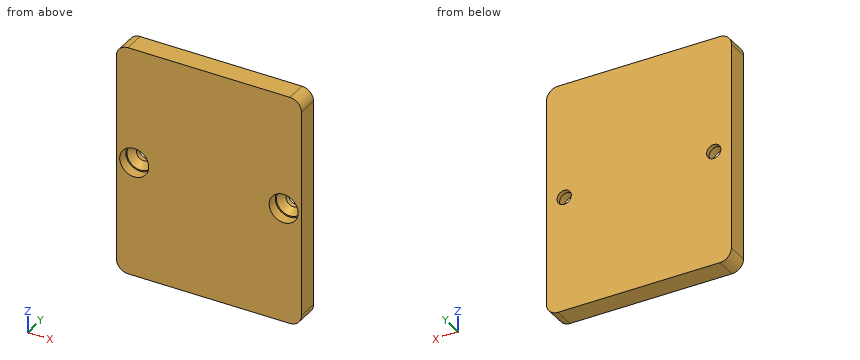
from build123d import *

# Parameters (mm, degrees)
SKETCH1_R                                       = 1.5
BOSS_EXTRUDE1_DEPTH                             = 2.5
CSK_FOR_M3_FLAT_HEAD_MACHINE_SCREW1_D           = 3.4
CSK_FOR_M3_FLAT_HEAD_MACHINE_SCREW1_DEPTH       = 10
CSK_FOR_M3_FLAT_HEAD_MACHINE_SCREW1_CSINK_D     = 6.3
CSK_FOR_M3_FLAT_HEAD_MACHINE_SCREW1_CSINK_ANGLE = 90
CSK_FOR_M3_FLAT_HEAD_MACHINE_SCREW1_TIP         = 1.021463052
BOSS_EXTRUDE2_START                             = 2.5
SKETCH4_R                                       = 3.45
BOSS_EXTRUDE2_DEPTH                             = 2.5


with BuildPart() as part:
    # Sketch1 → Boss-Extrude1 (new body)
    with BuildSketch(Plane(origin=(0, 0, 0), x_dir=(1, 0, 0), z_dir=(0, 1, 0))):
        with BuildLine():
            Line((-19.25, -27.5), (19.25, -27.5))
            ThreePointArc((19.25, -27.5), (21.194543648, -26.694543648), (22, -24.75))
            Line((22, -24.75), (22, 24.75))
            ThreePointArc((22, 24.75), (21.194543648, 26.694543648), (19.25, 27.5))
            Line((19.25, 27.5), (-19.25, 27.5))
            ThreePointArc((-19.25, 27.5), (-21.194543648, 26.694543648), (-22, 24.75))
            Line((-22, 24.75), (-22, -24.75))
            ThreePointArc((-22, -24.75), (-21.194543648, -26.694543648), (-19.25, -27.5))
        make_face()
        with Locations(Location((-17.78, 0, 0), (0, 0, 270))):
            Circle(SKETCH1_R, mode=Mode.SUBTRACT)
        with Locations(Location((17.78, 0, 0), (0, 0, 90))):
            Circle(SKETCH1_R, mode=Mode.SUBTRACT)
    extrude(amount=BOSS_EXTRUDE1_DEPTH)

    # CSK for M3 Flat Head Machine Screw1
    with Locations(Plane(origin=(0, 0, 0), x_dir=(-1, 0, 0), z_dir=(0, -1, 0))):
        with Locations((-17.78, 0), (17.78, 0)):
            CounterSinkHole(CSK_FOR_M3_FLAT_HEAD_MACHINE_SCREW1_D / 2, CSK_FOR_M3_FLAT_HEAD_MACHINE_SCREW1_CSINK_D / 2, depth=CSK_FOR_M3_FLAT_HEAD_MACHINE_SCREW1_DEPTH, counter_sink_angle=CSK_FOR_M3_FLAT_HEAD_MACHINE_SCREW1_CSINK_ANGLE)
            with Locations((0, 0, -(CSK_FOR_M3_FLAT_HEAD_MACHINE_SCREW1_DEPTH + CSK_FOR_M3_FLAT_HEAD_MACHINE_SCREW1_TIP / 2))):  # 118° drill point
                Cone(0, CSK_FOR_M3_FLAT_HEAD_MACHINE_SCREW1_D / 2, CSK_FOR_M3_FLAT_HEAD_MACHINE_SCREW1_TIP, mode=Mode.SUBTRACT)

    # Sketch4 → Boss-Extrude2 (add)
    with BuildSketch(Plane.XZ.offset(BOSS_EXTRUDE2_START)):
        with BuildLine():
            Line((-22, 24.75), (-22, -24.75))
            ThreePointArc((-22, -24.75), (-21.194543648, -26.694543648), (-19.25, -27.5))
            Line((-19.25, -27.5), (19.25, -27.5))
            ThreePointArc((19.25, -27.5), (21.194543648, -26.694543648), (22, -24.75))
            Line((22, -24.75), (22, 24.75))
            ThreePointArc((22, 24.75), (21.194543648, 26.694543648), (19.25, 27.5))
            Line((19.25, 27.5), (-19.25, 27.5))
            ThreePointArc((-19.25, 27.5), (-21.194543648, 26.694543648), (-22, 24.75))
        make_face()
        with Locations(Location((-17.78, 0, 0), (0, 0, 270))):
            Circle(SKETCH4_R, mode=Mode.SUBTRACT)
        with Locations(Location((17.78, 0, 0), (0, 0, 270))):
            Circle(SKETCH4_R, mode=Mode.SUBTRACT)
    extrude(amount=-BOSS_EXTRUDE2_DEPTH)


solid = part.part
Design review of the part built by this model. Coordinates are the model's own, in mm. Round coordinates to 2 decimals unless told otherwise and drop trailing zeros. Loops run counter-clockwise (first coordinate to the right, second up) from the corner with the lowest first, then second, coordinate; pieces in that order, holes last. Notation, with made-up numbers: M 62,-32 L 92,-32 A30 cw 92,-3 Z; hole C 74.5,74 d10. An arc over 180 degrees is marked long. Answer as a JSON object with one key per item and string values.
Item 1: We need section A-A on z = 0. Give the boundary of the cut face in (x, y).
Answer sheet:
{"outline": "M -22,-2.5 L -21.23,-2.5 L -21.23,0 L -20.93,0 L -19.48,1.45 L -19.48,2.5 L -22,2.5 Z; M -16.08,1.45 L -14.63,0 L -14.33,0 L -14.33,-2.5 L 14.33,-2.5 L 14.33,0 L 14.63,0 L 16.08,1.45 L 16.08,2.5 L -16.08,2.5 Z; M 19.48,1.45 L 20.93,0 L 21.23,0 L 21.23,-2.5 L 22,-2.5 L 22,2.5 L 19.48,2.5 Z"}
Item 2: We need section B-B on x = -17.78. Give the boundary of the cut face in (y, z), and give its area (3 significant figures).
Answer sheet:
{"outline": "M -2.5,-27.5 L 2.5,-27.5 L 2.5,-1.7 L 1.45,-1.7 L 0,-3.15 L 0,-3.45 L -2.5,-3.45 Z; M -2.5,3.45 L 0,3.45 L 0,3.15 L 1.45,1.7 L 2.5,1.7 L 2.5,27.5 L -2.5,27.5 Z", "area": "247 mm^2"}
Item 3: Clearance check with flat-ended pins moving along their axes: P1, Ø3.5, axis at x = -18.5, z = 0, coming from the -Y side; P2, Ø4, axis at x = -17.78, z = 0, coming from the -Y side. State where each tip first meets the part, or that it passes through.
Answer sheet:
{"P1": "stops at y = 0.68", "P2": "stops at y = 1.15"}
Item 4: We need section C-C on y = -1.05. Give the boundary of the cut face in (x, z).
Answer sheet:
{"outline": "M -22,-24.75 A2.75 ccw -19.25,-27.5 L 19.25,-27.5 A2.75 ccw 22,-24.75 L 22,24.75 A2.75 ccw 19.25,27.5 L -19.25,27.5 A2.75 ccw -22,24.75 Z; hole C -17.78,0 d6.9; hole C 17.78,0 d6.9"}
Item 5: Wall thickness on L1, parallel to X at y = -1.3, z = 0; L2, parallel to X at y = -1.55, z = 2; L3, parallel to Z at x = -17.78, y = 2.25: over which ranges is each line inside the solid? List them lowest first. Write a range as from..to.
Answer sheet:
{"L1": "x = -22..-21.23, -14.33..14.33, 21.23..22", "L2": "x = -22..-20.59, -14.97..14.97, 20.59..22", "L3": "z = -27.5..-1.7, 1.7..27.5"}
